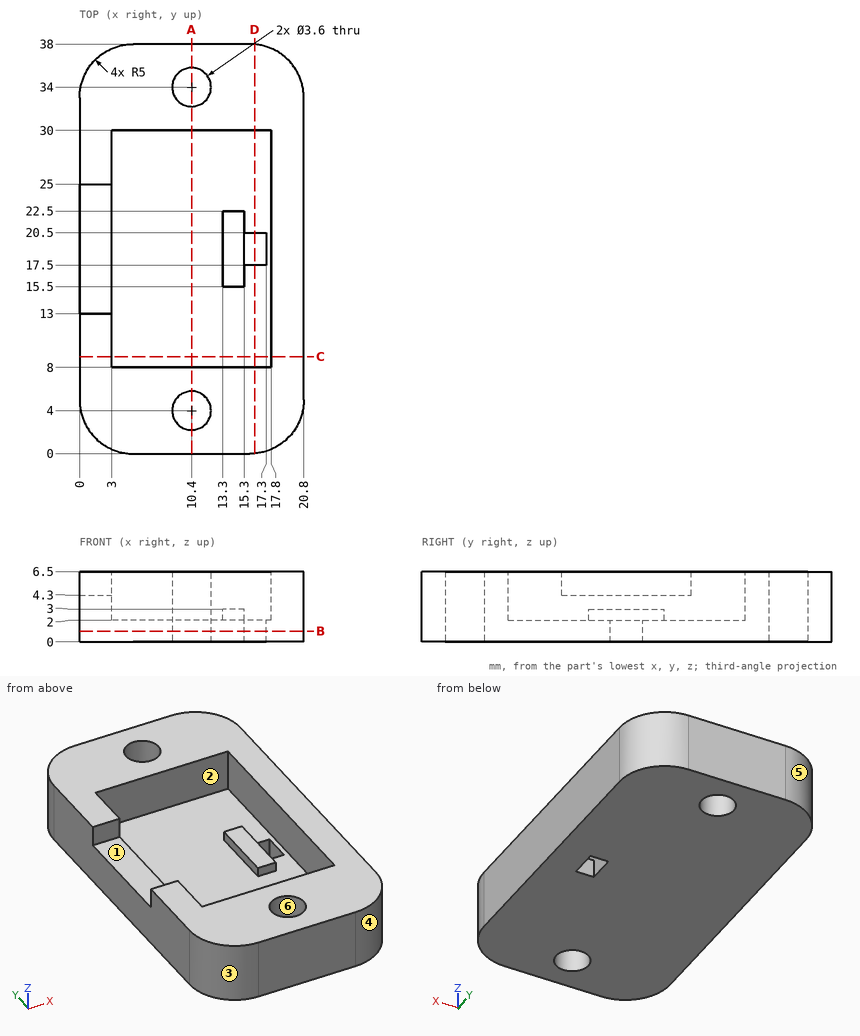
Answer from the drawing. Dimensions are ordinates in mm from the lowest x, y and z of the part. A direction names the side the tool comes from. Give positions to 0.01 mm unless a question says otherwise; leave off trailing zeros. Loops run counter-clockwise (first coordinate to the right, second up) from the corner with the lowest first, then second, coordinate; pieces in that order, holes last.
Item 1: A cutting plane is placed at C-C (y = 9). Give the vertices of the cut face in (x, z).
Derived:
outline: (0, 0) - (20.8, 0) - (20.8, 6.5) - (17.8, 6.5) - (17.8, 2) - (3, 2) - (3, 6.5) - (0, 6.5) - close
Item 2: Find the intervals of material crossed by line 1 along Y through (x, z) = (14.75, 2.25); line 2 along Y through (x, z) = (10.4, 4.75); line 3 along Y through (x, z) = (15, 5.75), in increasing order.
Derived:
line 1: y = 0 to 8, 15.5 to 22.5, 30 to 38
line 2: y = 0 to 2.2, 5.8 to 8, 30 to 32.2, 35.8 to 38
line 3: y = 0 to 8, 30 to 38
Item 3: A cutting plane is placed at B-B (z = 1). Give the vertices of the cut face in (x, y), then the cut area to 3 significant figures.
Derived:
outline: (0, 5) arc R5 ccw to (5, 0) - (15.8, 0) arc R5 ccw to (20.8, 5) - (20.8, 33) arc R5 ccw to (15.8, 38) - (5, 38) arc R5 ccw to (0, 33) - close; hole circle Ø3.6 at (10.4, 4); hole circle Ø3.6 at (10.4, 34); hole (15.3, 17.5) - (17.3, 17.5) - (17.3, 20.5) - (15.3, 20.5) - close
area: 743 mm2
Item 4: A tool of negligible diameter and unlimited length cuts with its end or side. For the marked faces 1, 2 and 3, from which of +Z, -Z, +X, -X, +Y, -Y can it reach the whole face along a straight path? Write none if from no direction.
Derived:
face 1: +Z, -X
face 2: +Z
face 3: +Z, -Z, -X, -Y
Item 5: Each of these flat-tipped pins is pushed along its axis until it touches: pin 1 Ø1.1 at (x, z) = (2, 5.5) entering from +Y; pin 2 Ø0.6 at (x, y) = (14, 17.5) entering from +Z; pin 3 Ø2.5 at (x, z) = (1, 5.5) entering from -Y. Where does it stop, or does it pass through?
Derived:
pin 1: stops at y = 37.36
pin 2: stops at z = 3
pin 3: stops at y = 0.82
Item 6: A cutting plane is placed at D-D (x = 16.25). Give the vertices of the cut face in (y, z), then the cut area to 3 significant figures.
Derived:
outline: (0.02, 0) - (17.5, 0) - (17.5, 2) - (8, 2) - (8, 6.5) - (0.02, 6.5) - close; (20.5, 0) - (37.98, 0) - (37.98, 6.5) - (30, 6.5) - (30, 2) - (20.5, 2) - close
area: 142 mm2
Item 7: Determine the mould class of the marked faces 4, 5 and 6 for opening direction Y: +Y half, -Y half, draft (parallel to the pull), parting line (faces both ways), or undercut.
Derived:
face 4: -Y half
face 5: +Y half
face 6: undercut
Item 8: A cutting plane is placed at A-A (x = 10.4). Give the vertices of the cut face in (y, z), then the cut area to 3 significant figures.
Derived:
outline: (0, 0) - (2.2, 0) - (2.2, 6.5) - (0, 6.5) - close; (5.8, 0) - (32.2, 0) - (32.2, 6.5) - (30, 6.5) - (30, 2) - (8, 2) - (8, 6.5) - (5.8, 6.5) - close; (35.8, 0) - (38, 0) - (38, 6.5) - (35.8, 6.5) - close
area: 101 mm2
